from build123d import *

# Parameters (mm, degrees)
F0_R     = 12.7
F0_R_2   = 11.2
F1_DEPTH = 162.5
F2_R     = 4
F3_DEPTH = 175
F4_R     = 11.2
F5_DEPTH = 10
F6_R     = 11.2
F7_DEPTH = 10


with BuildPart() as f1:
    # F0 (on Right) → F1 (new body, symmetric)
    with BuildSketch(Plane.YZ):
        Circle(F0_R)
        Circle(F0_R_2, mode=Mode.SUBTRACT)
    extrude(amount=F1_DEPTH, both=True)



with BuildPart() as f3:
    # F2 (on Right) → F3 (new body, symmetric)
    with BuildSketch(Plane.YZ):
        Circle(F2_R)
    extrude(amount=F3_DEPTH, both=True)


with BuildPart() as f1_1:
    add(f1.part)

    add(f3.part)  # F5 merges F3
    # F4 (on face) → F5 (join)
    with BuildSketch(Plane.YZ.offset(162.5)):
        Circle(F4_R)
    extrude(amount=-F5_DEPTH)

    # F6 (on face) → F7 (join)
    with BuildSketch(Plane(origin=(-162.5, 0, 0), x_dir=(0, -1, 0), z_dir=(-1, 0, 0))):
        Circle(F6_R)
    extrude(amount=-F7_DEPTH)


solid = f1_1.part
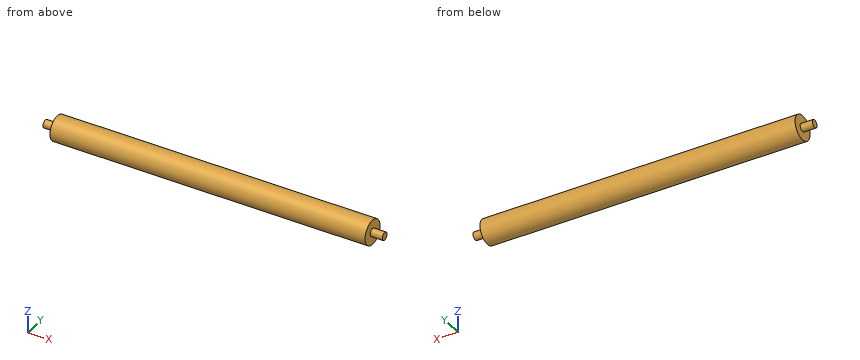
The model under review builds one solid part; all positions refer to its coordinate system, in mm. Coordinates: 2 decimals unless noted, no trailing zeros. Order: outer loops, then holes, each group sorted by start corner. A loop starts at its lowest first (then second) coordinate and runs counter-clockwise, first axis right, second up. Notation, with made-up numbers: (-7, 35.25) -> (27, 35.25) arc R5 cw to (27, 42.25) -> close; hole circle Ø7 at (57.25, -10). An arc over 180 degrees is marked (long way). Answer in a Markdown table with one row per item.
(1) Insertion check: pin 1 (4 mm diameter, centred on x = 75, y = 10, fed in from +Z); pin 2 (1 mm diameter, centred on x = 46, z = 10, fed in from -Y); pin 3 (12 mm diameter, centred on y = -3.5, z = -8.5, fed in from +X); pin 4 (1.5 mm diameter, centred on x = -55.5, y = -6.5, fed in from +Z). Each pin has a flat end and moves straight along its axis. Give the tip position at first contact, or say it passes through.
Answers:
| item | result |
|---|---|
| pin 1 | z = 9.86 |
| pin 2 | y = -8.43 |
| pin 3 | x = 175 |
| pin 4 | z = 11.32 |
(2) Consider section A-A (y = 0). Write out the cut boundary in (x, z).
Answers:
| item | result |
|---|---|
| outline | (-175, -4) -> (-162.5, -4) -> (-162.5, -12.7) -> (162.5, -12.7) -> (162.5, -4) -> (175, -4) -> (175, 4) -> (162.5, 4) -> (162.5, 12.7) -> (-162.5, 12.7) -> (-162.5, 4) -> (-175, 4) -> close; hole (-152.5, -11.2) -> (152.5, -11.2) -> (152.5, -4) -> (-152.5, -4) -> close; hole (-152.5, 4) -> (152.5, 4) -> (152.5, 11.2) -> (-152.5, 11.2) -> close |
(3) Wall thickness on line 1 along Z through (x, y) = (4, 0); line 2 along Y through (x, z) = (12.5, 2.75); line 3 along Z through (x, y) = (52, 3.5): over which ranges is each line inside the solid? List them lowest first.
Answers:
| item | result |
|---|---|
| line 1 | -12.7 to -11.2, -4 to 4, 11.2 to 12.7 |
| line 2 | -12.4 to -10.86, -2.9 to 2.9, 10.86 to 12.4 |
| line 3 | -12.21 to -10.64, -1.94 to 1.94, 10.64 to 12.21 |
(4) Consider section C-C (x = -78). Write out the cut boundary in (y, z), plus the area to 3 significant figures.
Answers:
| item | result |
|---|---|
| outline | circle Ø25.4 at (0, 0); circle Ø8 at (0, 0); hole circle Ø22.4 at (0, 0) |
| area | 163 mm² |
